```python
from build123d import *

# Parameters (mm, degrees)
CHAMFER3_SIZE = 0.2
FILLET2_R     = 1


with BuildPart() as part:
    # Sketch1 → Revolve1 (revolve)
    with BuildSketch(Plane(origin=(0, 0, 0), x_dir=(1, 0, 0), z_dir=(0, 1, 0)), mode=Mode.PRIVATE) as revolve1_sk:
        Polygon((4, 0), (2.5, 0), (2.5, 6), (0, 6), (0, 9), (10.75, 9), (10.75, 7.762245205), (5.75, 7.762245205), (5.75, 7), (4, 7), align=None)
    revolve(revolve1_sk.sketch.rotate(Axis((0, 0, -9.865928584), (0, 0, 1)), 180), axis=Axis((0, 0, -9.865928584), (0, 0, 1)))

    # Chamfer3
    chamfer3_edges = [part.edges().sort_by_distance(p)[0] for p in [
        (4, 0, 0),
    ]]
    chamfer(chamfer3_edges, length=CHAMFER3_SIZE)

    # Fillet2
    fillet2_edges = [part.edges().sort_by_distance(p)[0] for p in [
        (10.75, 0, -9),
    ]]
    fillet(fillet2_edges, radius=FILLET2_R)


solid = part.part
```
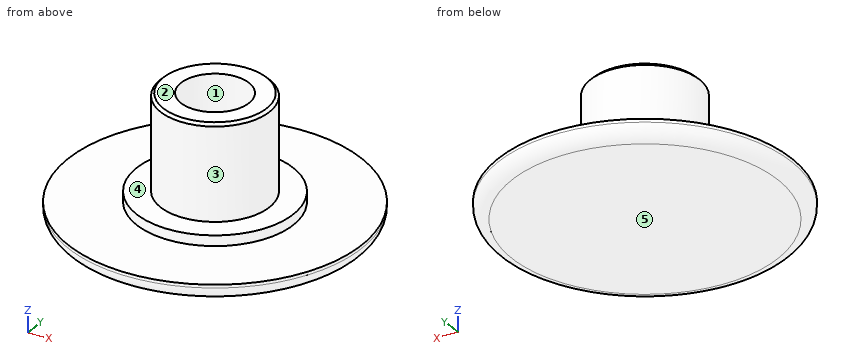
Geometry: final body of the model. Coordinates: model frame, mm. Face numbers are marked on the shaded views. A direction names the side the tool comes from. Give positions to 0.01 mm unless a question says otherwise; leave off trailing zeros. Loops run counter-clockwise (first coordinate to the right, second up) from the corner with the lowest first, then second, coordinate; pieces in that order, holes last. Notation, with made-up numbers: (83.5, 0) -> (93.5, 0) arc R19 cw to (93.5, 13) -> close; hole circle Ø1 at (43.5, -3). An arc over 180 degrees is marked (long way). Return JSON: item names as keys, results as strings.
Item 1: Mould query, pull axis Y, two halves, no side actions, for the marked faces 1, 2 and 3. Classes: released by +Y, released by -Y, zero draft, split by the parting line, or undercut.
Filled in:
{"face 1": "undercut", "face 2": "zero draft", "face 3": "split by the parting line"}
Item 2: Access query for the marked faces 4 and 5. Directions: +Z, -Z, +X, -X, +Y, -Y. A direction counts if a zero-diameter tool reaches every point of the face in a straight line with its end or side. Return the directions, or none.
Filled in:
{"face 4": "+Z", "face 5": "-Z, +X, -X, +Y, -Y"}
Item 3: Line query: line 1 (Y direction, x = 0, z = -1.7); line 2 (Z direction, x = 3, y = 3.5); line 3 (Z direction, x = 6.5, y = 3). Output: solid intervals per line, ascending.
Filled in:
{"line 1": "-4 to -2.5, 2.5 to 4", "line 2": "-9 to -7", "line 3": "-9 to -7.76"}
Item 4: Section A-A, the plane z = -0.75. Output: boundary loops of the cut face in (x, y), plus the area to 3 significant figures.
Filled in:
{"outline": "circle Ø8 at (0, 0); hole circle Ø5 at (0, 0)", "area": "30.6 mm^2"}
Item 5: Pin query (flat end, axial travel): P1, Ø3, axis at y = -6.5, z = -3, coming from the +X side; P2, Ø2.5, axis at x = 0.5, y = -0.5, coming from the +Z side; P3, Ø5, axis at x = -7.5, y = 0.5, coming from the +Z side; P4, Ø1, axis at y = 4.5, z = -7, coming from the -X side. Return the tip coordinate at first contact, or that it passes through.
Filled in:
{"P1": "through", "P2": "z = -6", "P3": "z = -7", "P4": "x = -4.13"}
Item 6: Section B-B, the plane y = 0. Output: boundary loops of the cut face in (x, z).
Filled in:
{"outline": "(-10.75, -8) arc R1 ccw to (-9.75, -9) -> (9.75, -9) arc R1 ccw to (10.75, -8) -> (10.75, -7.76) -> (5.75, -7.76) -> (5.75, -7) -> (4, -7) -> (4, -0.2) -> (3.8, 0) -> (2.5, 0) -> (2.5, -6) -> (-2.5, -6) -> (-2.5, 0) -> (-3.8, 0) -> (-4, -0.2) -> (-4, -7) -> (-5.75, -7) -> (-5.75, -7.76) -> (-10.75, -7.76) -> close"}
